Check sheet for the modelled part. Datum: model origin and axes. Units: mm. Give positions to 0.01 mm unless a question says otherwise; leave off trailing zeros. Loops run counter-clockwise (first coordinate to the right, second up) from the corner with the lowest first, then second, coordinate; pieces in that order, holes last. Notation, with made-up numbers: (28.25, 56) -> (50.25, 56) arc R13 ccw to (50.25, 79) -> close; hole circle Ø8 at (26.25, 67.5). An arc over 180 degrees is marked (long way). Answer as CSV lines item,"result". Start each with the question number.
(1) Material ranges on line 1 (Z direction, x = 9, y = 22); line 2 (X direction, y = 12.5, z = -1.5); line 3 (X direction, y = -8, z = -2.25), recorded low to high. Write a range as from..to.
(2) Section check B-B on y = 0. Enter the section's corners in (x, z) (3 decimals).
(3) Gauge pin test, flat ends, axial feed: pin 1 Ø1.3 at (x, z) = (-19, -2) entering from +Y; pin 2 Ø1.2 at (x, z) = (19, 3.5) entering from +Y; pin 3 Ø3 at (x, z) = (19.5, 4) entering from -Y; pin 4 Ø2.5 at (x, y) = (-15.41, 12.75) entering from +Z (3 decimals). Record the tip position at first contact, or that the pin passes through.
(4) Section check C-C on x = 0. Enter the section's corners in (y, z) (3 decimals), plus the area to 3 significant figures.
(5) Section check D-D on y = 5. Enter the section's corners in (x, z) (3 decimals).
(6) Section check A-A on z = 7.25. Enter the section's corners in (x, y) (3 decimals).
from build123d import *

# Parameters (mm, degrees)
SKETCH1_R           = 24.875
BOSS_EXTRUDE2_DEPTH = 3
SKETCH1_4_W         = 2.5
SKETCH1_4_H         = 13.6
BOSS_EXTRUDE3_DEPTH = 8.46
CUT_EXTRUDE1_DEPTH  = 2.5
SKETCH10_R          = 1.5
CUT_EXTRUDE3_DEPTH  = 4.95
SKETCH5_W           = 2.6
SKETCH5_H           = 11.7
CUT_EXTRUDE4_DEPTH  = 4.95


with BuildPart() as part:
    # Sketch1 → Boss-Extrude2 (new body)
    with BuildSketch(Plane.XY):
        Circle(SKETCH1_R)
    extrude(amount=-BOSS_EXTRUDE2_DEPTH)

    # Sketch1<4> → Boss-Extrude3 (add)
    with BuildSketch(Plane.XY):
        with Locations((19.005, 0)):
            Rectangle(SKETCH1_4_W, SKETCH1_4_H)
    extrude(amount=BOSS_EXTRUDE3_DEPTH)

    # Sketch4 → Cut-Extrude1 (cut)
    with BuildSketch(Plane(origin=(20.255, 0, 0), x_dir=(0, 0, -1), z_dir=(1, 0, 0))):
        with BuildLine():
            ThreePointArc((-0.931303911, -0.65), (-3.48591682, 0), (-0.931303911, 0.65))
            Line((-0.931303911, 0.65), (-0.931303911, 5.8))
            Line((-0.931303911, 5.8), (-8.46, 5.8))
            Line((-8.46, 5.8), (-8.46, -5.8))
            Line((-8.46, -5.8), (-0.931303911, -5.8))
            Line((-0.931303911, -5.8), (-0.931303911, -0.65))
        make_face()
    extrude(amount=-CUT_EXTRUDE1_DEPTH, mode=Mode.SUBTRACT)

    # Sketch10 → Cut-Extrude3 (cut)
    with BuildSketch(Plane.XY):
        with Locations((-15.409206931, 12.75144494)):
            Circle(SKETCH10_R)
        with Locations((-15.409206931, -11.899319199)):
            Circle(SKETCH10_R)
    extrude(amount=-CUT_EXTRUDE3_DEPTH, mode=Mode.SUBTRACT)

    # Sketch5 → Cut-Extrude4 (cut)
    with BuildSketch(Plane.XY):
        with Locations((-18.96, 0)):
            Rectangle(SKETCH5_W, SKETCH5_H)
    extrude(amount=-CUT_EXTRUDE4_DEPTH, mode=Mode.SUBTRACT)


solid = part.part
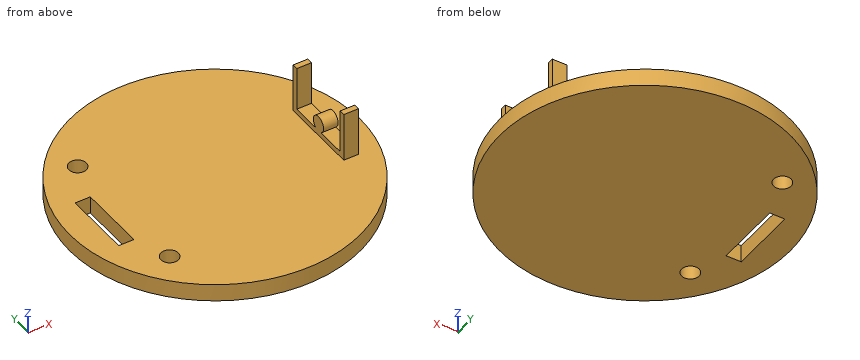
Working result:
1,line 1,"z = -3..0"
1,line 2,"x = -21.51..-16.89, -13.93..21.51"
1,line 3,"x = -23.55..23.55"
2,outline,"(-24.875, -3) -> (-20.26, -3) -> (-20.26, 0) -> (-24.875, 0) -> close; (-17.66, -3) -> (24.875, -3) -> (24.875, 0) -> (20.255, 0) -> (20.255, 3.486) -> (17.755, 3.486) -> (17.755, 0) -> (-17.66, 0) -> close"
3,pin 1,"stops at y = 16.79"
3,pin 2,"stops at y = 6.8"
3,pin 3,"stops at y = -6.8"
3,pin 4,"passes through"
4,outline,"(-24.875, -3) -> (24.875, -3) -> (24.875, 0) -> (-24.875, 0) -> close"
4,area,"149 mm^2"
5,outline,"(-24.367, -3) -> (-20.26, -3) -> (-20.26, 0) -> (-24.367, 0) -> close; (-17.66, -3) -> (24.367, -3) -> (24.367, 0) -> (20.255, 0) -> (20.255, 0.931) -> (17.755, 0.931) -> (17.755, 0) -> (-17.66, 0) -> close"
6,outline,"(17.755, -6.8) -> (20.255, -6.8) -> (20.255, -5.8) -> (17.755, -5.8) -> close; (17.755, 5.8) -> (20.255, 5.8) -> (20.255, 6.8) -> (17.755, 6.8) -> close"
